```python
from build123d import *

# Parameters (mm, degrees)
SKETCH_1_W          = 15
SKETCH_1_H          = 21.5
EXTRUDE_1_DEPTH     = 2
SKETCH_2_W          = 12.5
SKETCH_2_H          = 19
EXTRUDE_2_DEPTH     = 13.5
SKETCH_3_W          = 9.5
SKETCH_3_H          = 15
EXTRUDE_3_DEPTH     = 4
CUT_EXTRUDE_START   = -9.5
CUT_EXTRUDE_1_DEPTH = 9.5
SKETCH_6_W          = 3
SKETCH_6_H          = 1
EXTRUDE_1_2_DEPTH   = 7.5


# Read off the part's stored shape, not the designer's step: 切除-拉伸1
with BuildPart() as part:
    # 草图1 → Extrude 1 (new body)
    with BuildSketch(Plane.XY):
        Rectangle(SKETCH_1_W, SKETCH_1_H)
    extrude(amount=EXTRUDE_1_DEPTH)

    # 草图2 → 拉伸2 (add)
    with BuildSketch(Plane.XY.offset(2)):
        Rectangle(SKETCH_2_W, SKETCH_2_H)
    extrude(amount=EXTRUDE_2_DEPTH)

    # 草图3 → 拉伸3 (add)
    with BuildSketch(Plane(origin=(0, 0, 0), x_dir=(-1, 0, 0), z_dir=(0, 0, -1))):
        Rectangle(SKETCH_3_W, SKETCH_3_H)
    extrude(amount=EXTRUDE_3_DEPTH)

    # 切除-拉伸1 outline → 切除-拉伸1 (cut)
    with BuildSketch(Plane.ZY.offset(4.75).offset(CUT_EXTRUDE_START)):
        with BuildLine():
            Line((-4, -7.5), (-0.355698538, -7.5))
            add(Edge.make_bspline(
                [(-0.355698538, -7.5), (-0.354349182, -7.203584733), (-0.342893084, -4.687006069), (-0.90591647, 0.423075599), (-2.923742076, 4.765110149), (-4, 7.081043238)],
                knots=[0, 0, 0, 0, 0.058645761, 0.497905094, 1, 1, 1, 1], degree=3))
            Line((-4, 7.081043238), (-4, -7.5))
        make_face()
        with BuildLine():
            Line((-4, 7.5), (-4, 7.081043238))
            add(Edge.make_bspline(
                [(-4, 7.081043238), (-3.418318642, 7.19501669), (-2.098267317, 7.453664838), (-0.752663012, 7.483379257), (0, 7.5)],
                knots=[0, 0, 0, 0, 0.440650562, 1, 1, 1, 1], degree=3))
            Line((0, 7.5), (-4, 7.5))
        make_face()
    extrude(amount=CUT_EXTRUDE_1_DEPTH, mode=Mode.SUBTRACT)

    # 草图6 → Extrude 1 2 (add)
    with BuildSketch(Plane.XY.offset(15.5)):
        Rectangle(SKETCH_6_W, SKETCH_6_H)
    extrude(amount=EXTRUDE_1_2_DEPTH)


solid = part.part
```
Check sheet for the modelled part. Datum: model origin and axes. Units: mm. A direction names the side the tool comes from. Give positions to 0.01 mm unless a question says otherwise; leave off trailing zeros. Order: outer loops, then holes, each group sorted by start corner. A loop starts at its lowest first (then second) coordinate and runs counter-clockwise, first axis right, second up. Notation, with made-up numbers: (80, -4.75) -> (115, -4.75) arc R21 cw to (115, 19.25) -> close; hole circle Ø5 at (-36.5, 63). An arc over 180 degrees is marked (long way). Use CSV: the item, a comma, the result in double quotes. Start each with the question number.
1) Go/stop test with flat-tipped pins: P1, Ø2, axis at x = 4, y = -5, coming from the -Z side; P2, Ø0.5, axis at y = 0, z = 19, coming from the +X side; P3, Ø3.5, axis at x = 0.5, z = 18, coming from the +Y side; P4, Ø5, axis at y = -2, z = 2.5, coming from the +X side. Record where each tip stops, or that it passes through.
2) Set-up check for faces 1 (the face through (6.25, 0, 9)), 2 (the face through (0, 9.5, 9)), 3 (the face through (4.75, 3, -1)): record each of +Z, -Z, +X, -X, +Y, -Y from which the full face is reachable in a straight line by a thin tool's end or side.
3) Sectioned sample at C-C, the plane z = 13.25. Record the boundary of the cut face in (x, y), plus the area to 4 significant figures.
4) Sectioned sample at B-B, the plane z = 16. Record the boundary of the cut face in (x, y), plus the area to 3 significant figures.
5) Sectioned sample at A-A, the plane y = -8.5. Record the boundary of the cut face in (x, z).
6) Material ranges on line 1 (Y direction, x = -6, z = 5); line 2 (X direction, y = 5, z = 10); line 3 (Z direction, x = -5.5, y = 2.5), recorded low to high. Write a range as from..to.
Recorded:
1,P1,"z = -0.49"
1,P2,"x = 1.5"
1,P3,"y = 0.5"
1,P4,"x = 7.5"
2,face 1,"+Z, +X, +Y, -Y"
2,face 2,"+Z, +X, -X, +Y"
2,face 3,"-Z, +X, +Y, -Y"
3,outline,"(-6.25, -9.5) -> (6.25, -9.5) -> (6.25, 9.5) -> (-6.25, 9.5) -> close"
3,area,"237.5 mm2"
4,outline,"(-1.5, -0.5) -> (1.5, -0.5) -> (1.5, 0.5) -> (-1.5, 0.5) -> close"
4,area,"3.00 mm2"
5,outline,"(-7.5, 0) -> (7.5, 0) -> (7.5, 2) -> (6.25, 2) -> (6.25, 15.5) -> (-6.25, 15.5) -> (-6.25, 2) -> (-7.5, 2) -> close"
6,line 1,"-9.5..9.5"
6,line 2,"-6.25..6.25"
6,line 3,"0..15.5"
